Answer from the drawing. Dimensions are ordinates in mm from the lowest x, y and z of the part. Round coordinates to 2 decimals unless told otherwise and drop trailing zeros. Write each loop counter-clockwise with the first axis right and the second up, starting at its lowest first coordinate (ties: lowest second). Pieces come first, ordered by that corner, then holes. Notation, with made-up numbers: (-5, 26.5) - (25, 26.5) arc R8 ccw to (25, 40.5) - close; hole circle Ø8 at (69, 18.25). An arc over 180 degrees is marked (long way). Return JSON: item names as keys, results as strings. Group by question number.
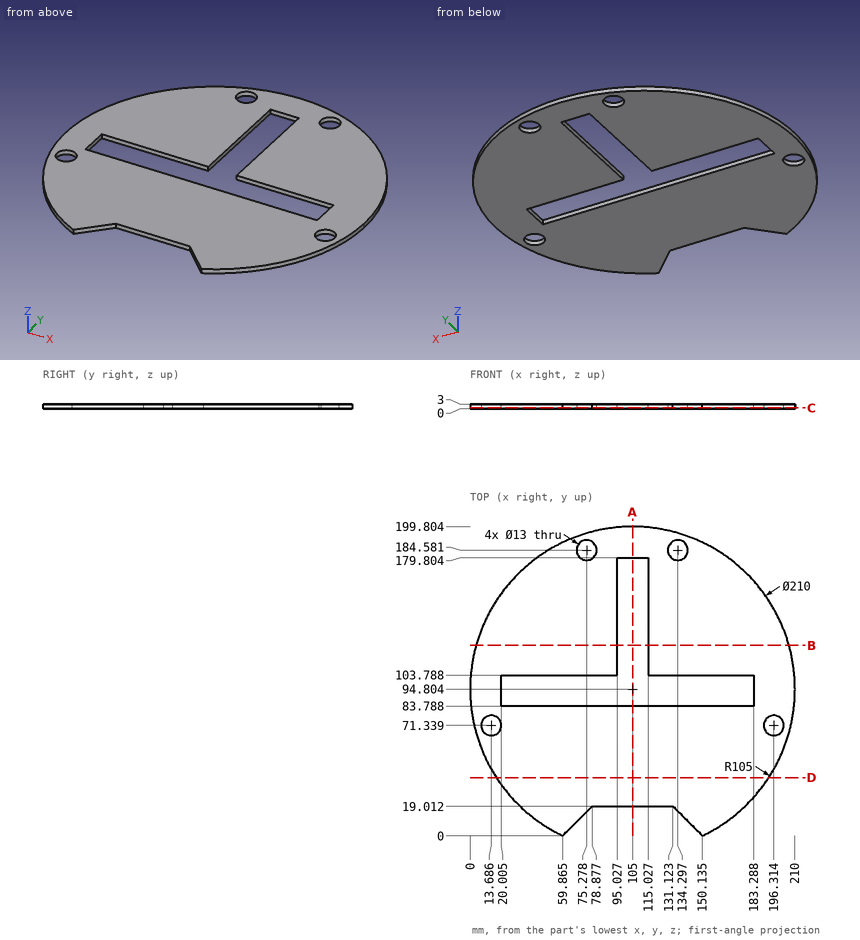
(1) Find section B-B (y = 123). Write down the section's boundary in (x, z), plus the area to 3 significant figures.
(2) Flat-ended cylindrical pins translate along their axes: pin 1 (1.5 mm diameter, centred on y = 91.5, z = 1, fed in from -X); pin 2 (0.9 mm diameter, centred on x = 145, z = 1.5, fed in from -Y) (1 decimal); pin 3 (0.9 mm diameter, centred on x = 110.5, z = 1.5, fed in from -Y). Find the tip coordinate at first contact, or state that the pin passes through.
(3) Consider line 1 (Y direction, x = 140, z = 1.9) (1 decimal); line 2 (X direction, y = 95.5, z = 1.25) (1 decimal); line 3 (Y direction, x = 166.5, z = 2.45). Determine where each line is inside the solid, lowest interval first.
(4) Find section C-C (z = 0.45). Write down the section's boundary in (x, y) (1 decimal), plus the area to 3 significant figures.
(5) Find section A-A (x = 105). Write down the section's boundary in (y, z) (1 decimal).
(6) Find section D-D (y = 37.5). Write down the section's boundary in (x, z) (1 decimal).
Check sheet entries:
{
 "1": {"outline": "(3.86, 0) - (95.03, 0) - (95.03, 3) - (3.86, 3) - close; (115.03, 0) - (206.14, 0) - (206.14, 3) - (115.03, 3) - close", "area": "547 mm^2"},
 "2": {"pin 1": "stops at x = 0.03", "pin 2": "stops at y = 4.7", "pin 3": "stops at y = 19.01"},
 "3": {"line 1": "y = 10.1 to 83.8, 103.8 to 181.5, 187.7 to 193.8", "line 2": "x = 0 to 20, 183.3 to 210", "line 3": "y = 9.7 to 83.79, 103.79 to 179.91"},
 "4": {"outline": "(59.9, 0) - (78.9, 19) - (131.1, 19) - (150.1, 0) arc R105 ccw (long way) to start; hole circle Ø13 at (13.7, 71.3); hole (20, 83.8) - (183.3, 83.8) - (183.3, 103.8) - (115, 103.8) - (115, 179.8) - (95, 179.8) - (95, 103.8) - (20, 103.8) - close; hole circle Ø13 at (75.3, 184.6); hole circle Ø13 at (134.3, 184.6); hole circle Ø13 at (196.3, 71.3)", "area": "27,300 mm^2"},
 "5": {"outline": "(19, 0) - (83.8, 0) - (83.8, 3) - (19, 3) - close; (179.8, 0) - (199.8, 0) - (199.8, 3) - (179.8, 3) - close"},
 "6": {"outline": "(17, 0) - (193, 0) - (193, 3) - (17, 3) - close"}
}
